For this review, take the finished solid that the model builds, in its own axes (mm). Coordinates: 2 decimals unless noted, no trailing zeros. Write each loop counter-clockwise with the first axis right and the second up, starting at its lowest first coordinate (ties: lowest second). Pieces come first, ordered by that corner, then holes. Notation, with made-up numbers: (-6, 30) - (19, 30) arc R29 cw to (19, 50) - close; hole circle Ø2 at (65, 69). An arc over 180 degrees is marked (long way). Use one line per item in the form item = value. Start each with the question number.
1) We need section D-D (x = 9). Give the boundary of the cut face in (y, z).
2) For L1, parallel to Y at x = -41, z = -0.15; L2, parallel to Y at x = 9, z = -0.45; L3, parallel to Y at x = -32.5, z = 1.8, list the stretches that pass through material, from the lowest coordinate up. Write a range as from..to.
3) We need section A-A (y = -41). Give the boundary of the cut face in (x, z), plus the area to 3 significant figures.
4) We need section C-C (y = 61). Give the boundary of the cut face in (x, z).
5) We need section B-B (z = 1.45). Count the separate pieces of the cut face and the enclosed holes in it, plus the area to 3 significant figures.
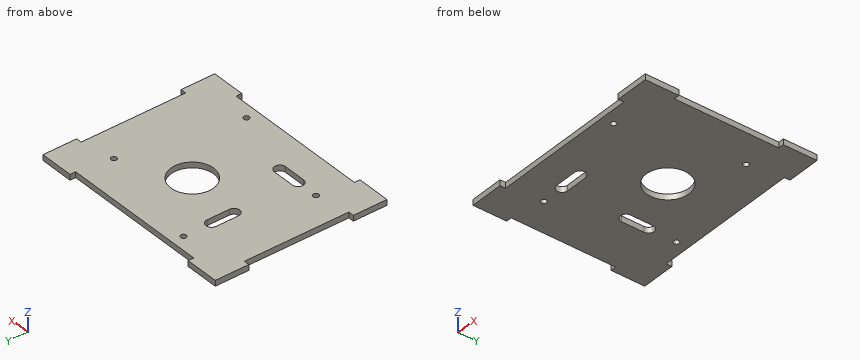
```python
from build123d import *

# Parameters (mm, degrees)
SKETCH_R   = 2.5
SKETCH_R_2 = 19
PAD_DEPTH  = 2.5


with BuildPart() as part:
    # Sketch → Pad (new body, symmetric)
    with BuildSketch(Plane.XY):
        Polygon((65.5, 76.5), (95.5, 76.5), (95.5, 46.5), (90.5, 46.5), (90.5, -46.5), (95.5, -46.5), (95.5, -76.5), (65.5, -76.5), (65.5, -71.5), (-65.5, -71.5), (-65.5, -76.5), (-95.5, -76.5), (-95.5, -46.5), (-90.5, -46.5), (-90.5, 46.5), (-95.5, 46.5), (-95.5, 76.5), (-65.5, 76.5), (-65.5, 71.5), (65.5, 71.5), align=None)
        with Locations((-61, -41)):
            Circle(SKETCH_R, mode=Mode.SUBTRACT)
        with Locations((41, -61)):
            Circle(SKETCH_R, mode=Mode.SUBTRACT)
        with Locations((9, 13)):
            Circle(SKETCH_R_2, mode=Mode.SUBTRACT)
        with Locations((61, 41)):
            Circle(SKETCH_R, mode=Mode.SUBTRACT)
        with Locations((-41, 61)):
            Circle(SKETCH_R, mode=Mode.SUBTRACT)
        with BuildLine():
            ThreePointArc((-36, 36), (-41, 41), (-46, 36))
            Line((-46, 36), (-46, 16))
            ThreePointArc((-46, 16), (-41, 11), (-36, 16))
            Line((-36, 36), (-36, 16))
        make_face(mode=Mode.SUBTRACT)
        with BuildLine():
            ThreePointArc((-41, -36), (-46, -41), (-41, -46))
            Line((-41, -46), (-21, -46))
            ThreePointArc((-21, -46), (-16, -41), (-21, -36))
            Line((-41, -36), (-21, -36))
        make_face(mode=Mode.SUBTRACT)
    extrude(amount=PAD_DEPTH, both=True)


solid = part.part
```
Determined:
q1.outline = (-71.5, -2.5) - (-6, -2.5) - (-6, 2.5) - (-71.5, 2.5) - close; (32, -2.5) - (71.5, -2.5) - (71.5, 2.5) - (32, 2.5) - close
q2.L1 = -71.5..-46, -36..11, 41..58.5, 63.5..71.5
q2.L2 = -71.5..-6, 32..71.5
q2.L3 = -71.5..-46, -36..71.5
q3.outline = (-90.5, -2.5) - (-63.5, -2.5) - (-63.5, 2.5) - (-90.5, 2.5) - close; (-58.5, -2.5) - (-46, -2.5) - (-46, 2.5) - (-58.5, 2.5) - close; (-16, -2.5) - (90.5, -2.5) - (90.5, 2.5) - (-16, 2.5) - close
q3.area = 730 mm²
q4.outline = (-95.5, -2.5) - (-43.5, -2.5) - (-43.5, 2.5) - (-95.5, 2.5) - close; (-38.5, -2.5) - (95.5, -2.5) - (95.5, 2.5) - (-38.5, 2.5) - close
q5.separate_pieces = 1
q5.enclosed_holes = 7
q5.area = 25,200 mm²
